Geometry check sheet. Reference: the model listing, model coordinates, mm. Round coordinates to 2 decimals unless told otherwise and drop trailing zeros. Order: outer loops, then holes, each group sorted by start corner. A loop starts at its lowest first (then second) coordinate and runs counter-clockwise, first axis right, second up.
(1) Sectioned sample at C-C (z = 31.5). Record the boundary of the cut face in (x, y).
(2) Go/stop test with flat-tipped pins: pin 1 (3 mm diameter, centred on x = -3, z = 39.95, fed in from +Y); pin 2 (0.5 mm diameter, centred on y = -1, z = 33, fed in from -X); pin 3 (0.5 mm diameter, centred on y = -1, z = 31.5, fed in from +X); pin 4 (4 mm diameter, centred on x = -16.83, z = 39.95, fed in from -Y). Record where each tip stops, or that it passes through.
(3) Sectioned sample at B-B (y = -1.1). Record the boundary of the cut face in (x, z) (3 decimals).
(4) Material ranges on line 1 along X through (y, z) = (-1.15, 6); line 2 along Z through (x, y) = (-18.25, -0.15); line 3 along Z through (x, y) = (-1, -1.15), recorded low to high.
(5) Sectioned sample at A-A (z = 1). Record the boundary of the cut face in (x, y), plus the area to 3 significant figures.
from build123d import *

# Parameters (mm, degrees)
F0_R     = 1.76
F1_DEPTH = 1.52


# Not quite as in the source:
# - a feature of the source that left no trace in its solid (it failed there, or was rolled back) is left out


with BuildPart() as f1:
    # F0 (on Front) → F1 (new body)
    with BuildSketch(Plane.XZ):
        Polygon((-13.44, 42.2827300502), (-19.83, 42.2827300502), (-19.83, 41.2284731865), (-19.83, 38.147136569), (-19.83, 37.9599481821), (-16.99, 35.5119891465), (-16.99, 29.9802143127), (-19.83, 25.8499481821), (-19.83, 25.4327300502), (-19.83, 22.0077300502), (-13.44, 22.0077300502), align=None)
        with Locations((-16.83, 39.9527300502)):
            Circle(F0_R, mode=Mode.SUBTRACT)
        with BuildLine():
            Line((-9.915, 42.2827300502), (-13.44, 42.2827300502))
            Line((-13.44, 42.2827300502), (-13.44, 22.0077300502))
            ThreePointArc((-13.44, 22.0077300502), (-12.4075514037, 24.5002814538), (-9.915, 25.5327300502))
            Line((-9.915, 25.5327300502), (-9.915, 42.2827300502))
        make_face()
        Polygon((-13.44, 22.0005065203), (-13.44, 22.0077300502), (-19.83, 22.0077300502), (-19.83, -8.4672699498), (-13.44, -8.4672699498), align=None)
        with BuildLine():
            Line((-6.39, 42.2827300502), (-9.915, 42.2827300502))
            Line((-9.915, 42.2827300502), (-9.915, 25.5327300502))
            ThreePointArc((-9.915, 25.5327300502), (-7.4224485963, 24.5002814538), (-6.39, 22.0077300502))
            Line((-6.39, 22.0077300502), (-6.39, 23.0757091194))
            Line((-6.39, 23.0757091194), (-6.39, 42.2827300502))
        make_face()
        Polygon((0, 42.2827300502), (-6.39, 42.2827300502), (-6.39, 23.0757091194), (-6.39, 22.0077300502), (-6.39, -8.4672699498), (0, -8.4672699498), (0, 25.4327300502), (0, 25.8499481821), (-2.84, 29.9802143127), (-2.84, 35.5119891465), (0, 37.9599481821), (0, 41.2284731865), align=None)
        with Locations((-3, 39.9527300502)):
            Circle(F0_R, mode=Mode.SUBTRACT)
        Polygon((-16.7724229395, -14.8872699498), (-13.44, -8.4672699498), (-19.83, -8.4672699498), align=None)
        Polygon((0, -8.4672699498), (-6.39, -8.4672699498), (-3.195, -14.8872699498), align=None)
    extrude(amount=F1_DEPTH)


solid = f1.part
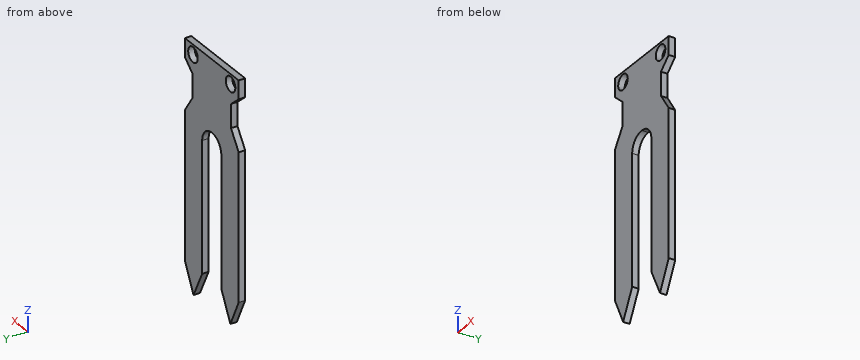
Answer below:
1. outline: (-16.99, -1.52) - (-2.84, -1.52) - (-2.84, 0) - (-16.99, 0) - close
2. pin 1: passes through
2. pin 2: stops at x = -16.99
2. pin 3: stops at x = -2.84
2. pin 4: stops at y = -1.52
3. outline: (-19.83, -8.467) - (-16.772, -14.887) - (-13.44, -8.467) - (-13.44, 22.008) arc R3.525 cw to (-6.39, 22.008) - (-6.39, -8.467) - (-3.195, -14.887) - (0, -8.467) - (0, 25.85) - (-2.84, 29.98) - (-2.84, 35.512) - (0, 37.96) - (0, 42.283) - (-19.83, 42.283) - (-19.83, 37.96) - (-16.99, 35.512) - (-16.99, 29.98) - (-19.83, 25.85) - close; hole circle Ø3.52 at (-16.83, 39.953); hole circle Ø3.52 at (-3, 39.953)
4. line 1: x = -19.83 to -13.44, -6.39 to 0
4. line 2: z = -11.78 to 28.15, 36.6 to 38.91, 40.99 to 42.28
4. line 3: z = -10.48 to 27.3, 37.1 to 42.28
5. outline: (-19.83, -1.52) - (-13.44, -1.52) - (-13.44, 0) - (-19.83, 0) - close; (-6.39, -1.52) - (0, -1.52) - (0, 0) - (-6.39, 0) - close
5. area: 19.4 mm2
